Design review of the part built by this model. Coordinates are the model's own, in mm. Face numbers are marked on the shaded views. A direction names the side the tool comes from. Coordinates: 2 decimals unless noted, no trailing zeros. Loops run counter-clockwise (first coordinate to the right, second up) from the corner with the lowest first, then second, coordinate; pieces in that order, holes last. Notation, with made-up numbers: M 42,89 L 80,89 A8 cw 80,95 Z; hole C 21,55 d1. An arc over 180 degrees is marked long. Put each result on its own line as item: value. Start each with the question number.
(1) Take a section at D-D, the plane x = -2.25. Give the boundary of the cut face in (y, z), then the cut area to 3 significant figures.
(2) Clearance check with flat-ended pins moving along their axes: pin 1 (2 mm diameter, centred on y = 11.5, z = 3, fed in from +X); pin 2 (1.5 mm diameter, centred on x = 1, z = 1, fed in from +Y); pin 3 (3 mm diameter, centred on x = -1.5, z = 1.5, fed in from +Y); pin 4 (1.5 mm diameter, centred on y = 11.5, z = 2.5, fed in from -X). State where each tip first meets the part, or that it passes through.
(3) Take a section at B-B, the plane x = 0. Give the boundary of the cut face in (y, z).
(4) For probe 1 along X at (y, z) = (0.75, 0); probe 2 along X at (y, z) = (11.75, 0); probe 3 along Y at (x, z) = (-1.25, -1.5), list the stretches that pass through material, from the lowest coordinate up. Write a range as [from, to].
(5) The part is to be moulded in two halves that separate along Z. For the marked faces 3, 4 and 5, say which applies: +Z half, -Z half, draft (parallel to the pull), parting line (faces both ways), or undercut.
(6) Take a section at C-C, the plane y = 7.5. Give the boundary of the cut face in (x, z).
(7) Take a section at A-A, the plane z = 0.25. Give the boundary of the cut face in (x, y), then the cut area to 3 significant figures.
(8) For the marked faces 1 and 2, list the 3-axis set-ups (+Z, -Z, +X, -X, +Y, -Y) from which the entire face can be reached by the end or side of a thin tool; tool diameter is ignored.
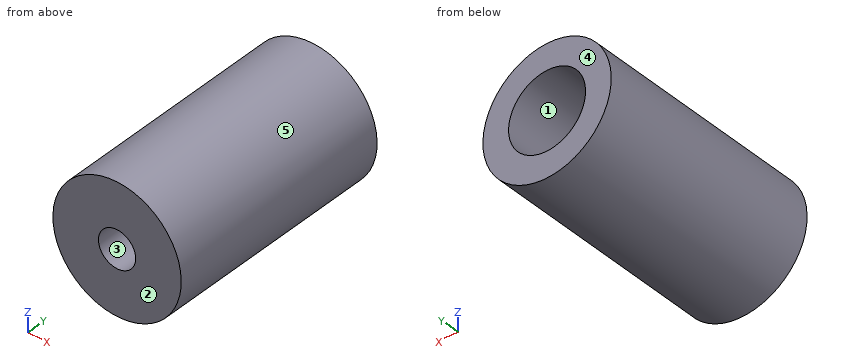
```python
from build123d import *

# Parameters (mm, degrees)
ESBO_O1_R                     = 5
RESSALTO_EXTRUS_O1_DEPTH      = 3
ESBO_O2_R                     = 5
ESBO_O2_R_2                   = 3
RESSALTO_EXTRUS_O2_DEPTH      = 15
FURO_COM_FOLGA_DE_M2_51_D     = 2.9
FURO_COM_FOLGA_DE_M2_51_DEPTH = 4
FURO_COM_FOLGA_DE_M2_51_TIP   = 0.871247898


with BuildPart() as part:
    # Esboço1 → Ressalto-extrusão1 (new body)
    with BuildSketch(Plane(origin=(0, 0, 0), x_dir=(1, 0, 0), z_dir=(0, 1, 0))):
        with Locations(Location((0, 0, 0), (0, 0, 270))):
            Circle(ESBO_O1_R)
    extrude(amount=RESSALTO_EXTRUS_O1_DEPTH)

    # Esboço2 → Ressalto-extrusão2 (add)
    with BuildSketch(Plane(origin=(0, 3, 0), x_dir=(1, 0, 0), z_dir=(0, 1, 0))):
        with Locations(Location((0, 0, 0), (0, 0, 270))):
            Circle(ESBO_O2_R)
        with Locations(Location((0, 0, 0), (0, 0, 270))):
            Circle(ESBO_O2_R_2, mode=Mode.SUBTRACT)
    extrude(amount=RESSALTO_EXTRUS_O2_DEPTH)

    # Furo com folga de M2.51
    with Locations(Plane(origin=(0, 0, 0), x_dir=(0, 0, -1), z_dir=(0, -1, 0))):
        with Locations((0, 0)):
            Hole(FURO_COM_FOLGA_DE_M2_51_D / 2, depth=FURO_COM_FOLGA_DE_M2_51_DEPTH)
            with Locations((0, 0, -(FURO_COM_FOLGA_DE_M2_51_DEPTH + FURO_COM_FOLGA_DE_M2_51_TIP / 2))):  # 118° drill point
                Cone(0, FURO_COM_FOLGA_DE_M2_51_D / 2, FURO_COM_FOLGA_DE_M2_51_TIP, mode=Mode.SUBTRACT)


solid = part.part
```
Computed values:
1. outline: M 0,-4.47 L 18,-4.47 L 18,-1.98 L 3,-1.98 L 3,1.98 L 18,1.98 L 18,4.47 L 0,4.47 Z
1. area: 101 mm^2
2. pin 1: stops at x = 4.58
2. pin 2: stops at y = 3
2. pin 3: stops at y = 18
2. pin 4: stops at x = -4.68
3. outline: M 0,-5 L 18,-5 L 18,-3 L 3,-3 L 3,-1.45 L 0,-1.45 Z; M 0,1.45 L 3,1.45 L 3,3 L 18,3 L 18,5 L 0,5 Z
4. probe 1: x = [-5, -1.45], [1.45, 5]
4. probe 2: x = [-5, -3], [3, 5]
4. probe 3: y = [0, 3]
5. face 3: undercut
5. face 4: draft
5. face 5: parting line
6. outline: C 0,0 d10; hole C 0,0 d6
7. outline: M -4.99,0 L -1.43,0 L -1.43,3 L -2.99,3 L -2.99,18 L -4.99,18 Z; M 1.43,0 L 4.99,0 L 4.99,18 L 2.99,18 L 2.99,3 L 1.43,3 Z
7. area: 81.5 mm^2
8. face 1: +Y
8. face 2: +Z, -Z, +X, -X, -Y
